Read the model definition and answer for the solid it produces. Units are mm, in the model's axes. A direction names the side the tool comes from. Give positions to 0.01 mm unless a question says otherwise; leave off trailing zeros. Order: outer loops, then holes, each group sorted by start corner. A loop starts at its lowest first (then second) coordinate and runs counter-clockwise, first axis right, second up.
Item 1: A cutting plane is placed at A-A (x = 0). Write down the section's boundary in (y, z), plus the area to 4 significant figures.
Item 2: A cutting plane is placed at B-B (y = -63). Write down the section's boundary in (x, z), plus the area to 3 significant figures.
Item 3: Which of the six approach directions +Z, -Z, +X, -X, +Y, -Y give full straight-line access (tool end or side, diameter ignored) to faces 4 (the face through (0, -37, 23.65)), 5 (the face through (0, -75, 26)), 6 (the face through (-15.81, 1.77, -14.75))?
Item 4: The mould has two halves that part along X. Classify faces 1 (the face through (-0.54, 2.46, 2.44)), 2 (the face through (27.5, -14, 25)), 3 (the face through (0, -34, 28.65)): +X half, -X half, draft (parallel to the pull), parting line (faces both ways), or undercut.
Item 5: A cutting plane is placed at D-D (y = -47.5). Write down the section's boundary in (x, z).
Item 6: Find the intervals of material crossed by line 1 along X through (y, z) = (1, -16); line 2 along Y through (x, z) = (15.5, 24.95); line 3 along Z through (x, y) = (15.5, 1), in increasing order.
Item 7: Given pin 1 Ø16.5 at (x, y) = (6, -36) entering from -Z; pin 2 Ø15.5 at (x, z) = (-7, -3.5) entering from -Y; pin 3 Ø4.5 at (x, y) = (0, -47.5) entering from -Z, each flat-ended and moving along its own axis, determine where each tip first touches the part or whether it passes through.
Item 8: A cutting plane is placed at C-C (z = 0). Write down the section's boundary in (x, y).
from build123d import *

# Parameters (mm, degrees)
SKETCH1_W                                         = 55
SKETCH1_H                                         = 57.3
SKETCH1_R                                         = 2.5
BOSS_EXTRUDE1_DEPTH                               = 5
SKETCH2_W                                         = 55
SKETCH2_H                                         = 5
BOSS_EXTRUDE2_DEPTH                               = 75
CUT_EXTRUDE1_REACH                                = 59.3
CUT_EXTRUDE2_REACH                                = 7
CUT_EXTRUDE3_REACH                                = 59.3
SKETCH5_R                                         = 2.5
CUT_EXTRUDE4_REACH                                = 59.3
SKETCH6_R                                         = 2.5
CUT_EXTRUDE5_REACH                                = 7
CSK_FOR_M2_5_FLAT_HEAD_MACHINE_SCREW1_D           = 2.9
CSK_FOR_M2_5_FLAT_HEAD_MACHINE_SCREW1_DEPTH       = 5
CSK_FOR_M2_5_FLAT_HEAD_MACHINE_SCREW1_CSINK_D     = 5.5
CSK_FOR_M2_5_FLAT_HEAD_MACHINE_SCREW1_CSINK_ANGLE = 90
F_6_40_TAPPED_HOLE1_D                             = 2.8702
F_6_40_TAPPED_HOLE1_DEPTH                         = 3.5
F_6_40_TAPPED_HOLE1_TIP                           = 0.862295074


with BuildPart() as part:
    # Sketch1 → Boss-Extrude1 (new body)
    with BuildSketch(Plane(origin=(0, 0, 0), x_dir=(1, 0, 0), z_dir=(0, 1, 0))):
        Rectangle(SKETCH1_W, SKETCH1_H)
        Circle(SKETCH1_R, mode=Mode.SUBTRACT)
    extrude(amount=BOSS_EXTRUDE1_DEPTH)

    # Sketch2 → Boss-Extrude2 (add)
    with BuildSketch(Plane.XZ):
        with Locations((0, 26.15)):
            Rectangle(SKETCH2_W, SKETCH2_H)
        with Locations((0, -26.15)):
            Rectangle(SKETCH2_W, SKETCH2_H)
    extrude(amount=BOSS_EXTRUDE2_DEPTH)

    # Sketch3 → Cut-Extrude1 (cut, up to next)
    with BuildSketch(Plane.XY.offset(28.65), mode=Mode.PRIVATE) as cut_extrude1_sk1:
        Polygon((-27.5, -75), (-17.5, -75), (-27.5, -65), align=None)
    cut_extrude1_tool1 = extrude(cut_extrude1_sk1.sketch, amount=-CUT_EXTRUDE1_REACH, mode=Mode.PRIVATE) & part.part
    add(cut_extrude1_tool1.solids().sort_by_distance((-24.166667, -71.666667, 28.65))[0], mode=Mode.SUBTRACT)
    # Sketch3 → Cut-Extrude1 (cut, up to next)
    with BuildSketch(Plane.XY.offset(28.65), mode=Mode.PRIVATE) as cut_extrude1_sk2:
        Polygon((27.5, -75), (27.5, -65), (17.5, -75), align=None)
    cut_extrude1_tool2 = extrude(cut_extrude1_sk2.sketch, amount=-CUT_EXTRUDE1_REACH, mode=Mode.PRIVATE) & part.part
    add(cut_extrude1_tool2.solids().sort_by_distance((24.166667, -71.666667, 28.65))[0], mode=Mode.SUBTRACT)

    # Sketch4 → Cut-Extrude2 (cut, up to next)
    with BuildSketch(Plane.XY.offset(-23.65), mode=Mode.PRIVATE) as cut_extrude2_sk1:
        Polygon((-27.5, -65), (-27.5, -75), (-17.5, -75), align=None)
    cut_extrude2_tool1 = extrude(cut_extrude2_sk1.sketch, amount=-CUT_EXTRUDE2_REACH, mode=Mode.PRIVATE) & part.part
    add(cut_extrude2_tool1.solids().sort_by_distance((-24.166667, -71.666667, -23.65))[0], mode=Mode.SUBTRACT)
    # Sketch4 → Cut-Extrude2 (cut, up to next)
    with BuildSketch(Plane.XY.offset(-23.65), mode=Mode.PRIVATE) as cut_extrude2_sk2:
        Polygon((27.5, -65), (17.5, -75), (27.5, -75), align=None)
    cut_extrude2_tool2 = extrude(cut_extrude2_sk2.sketch, amount=-CUT_EXTRUDE2_REACH, mode=Mode.PRIVATE) & part.part
    add(cut_extrude2_tool2.solids().sort_by_distance((24.166667, -71.666667, -23.65))[0], mode=Mode.SUBTRACT)

    # Sketch5 → Cut-Extrude3 (cut, up to next)
    with BuildSketch(Plane.XY.offset(28.65), mode=Mode.PRIVATE) as cut_extrude3_sk1:
        with Locations((0, -47.5)):
            Circle(SKETCH5_R)
    cut_extrude3_tool1 = extrude(cut_extrude3_sk1.sketch, amount=-CUT_EXTRUDE3_REACH, mode=Mode.PRIVATE) & part.part
    add(cut_extrude3_tool1.solids().sort_by_distance((0, -47.5, 28.65))[0], mode=Mode.SUBTRACT)

    # Sketch6 → Cut-Extrude4 (cut, up to next)
    with BuildSketch(Plane(origin=(0, 0, -28.65), x_dir=(-1, 0, 0), z_dir=(0, 0, -1)), mode=Mode.PRIVATE) as cut_extrude4_sk1:
        with Locations((0, -47.5)):
            Circle(SKETCH6_R)
    cut_extrude4_tool1 = extrude(cut_extrude4_sk1.sketch, amount=-CUT_EXTRUDE4_REACH, mode=Mode.PRIVATE) & part.part
    add(cut_extrude4_tool1.solids().sort_by_distance((0, -47.5, -28.65))[0], mode=Mode.SUBTRACT)

    # Sketch7 → Cut-Extrude5 (cut, up to next)
    with BuildSketch(Plane.XY.offset(-23.65), mode=Mode.PRIVATE) as cut_extrude5_sk1:
        Polygon((-27.5, 0), (27.5, 0), (27.5, -65), (17.5, -75), (-17.5, -75), (-27.5, -65), align=None)
    cut_extrude5_tool1 = extrude(cut_extrude5_sk1.sketch, amount=-CUT_EXTRUDE5_REACH, mode=Mode.PRIVATE) & part.part
    add(cut_extrude5_tool1.solids().sort_by_distance((0, -36.651139, -23.65))[0], mode=Mode.SUBTRACT)

    # CSK for M2.5 Flat Head Machine Screw1
    with Locations(Plane.XY.offset(28.65)):
        with Locations((-15.5, -32), (15.5, -32), (-15.5, -63), (15.5, -63)):
            CounterSinkHole(CSK_FOR_M2_5_FLAT_HEAD_MACHINE_SCREW1_D / 2, CSK_FOR_M2_5_FLAT_HEAD_MACHINE_SCREW1_CSINK_D / 2, depth=CSK_FOR_M2_5_FLAT_HEAD_MACHINE_SCREW1_DEPTH, counter_sink_angle=CSK_FOR_M2_5_FLAT_HEAD_MACHINE_SCREW1_CSINK_ANGLE)

    # #6-40 Tapped Hole1
    with Locations(Plane(origin=(0, 0, 0), x_dir=(-1, 0, 0), z_dir=(0, -1, 0))):
        with Locations((-15.5, 16.15), (15.5, 16.15)):
            Hole(F_6_40_TAPPED_HOLE1_D / 2, depth=F_6_40_TAPPED_HOLE1_DEPTH)
            with Locations((0, 0, -(F_6_40_TAPPED_HOLE1_DEPTH + F_6_40_TAPPED_HOLE1_TIP / 2))):  # 118° drill point
                Cone(0, F_6_40_TAPPED_HOLE1_D / 2, F_6_40_TAPPED_HOLE1_TIP, mode=Mode.SUBTRACT)


solid = part.part
Response values:
1. outline: (-75, 23.65) - (-50, 23.65) - (-50, 28.65) - (-75, 28.65) - close; (-45, 23.65) - (0, 23.65) - (0, 2.5) - (5, 2.5) - (5, 28.65) - (-45, 28.65) - close; (0, -28.65) - (5, -28.65) - (5, -2.5) - (0, -2.5) - close
1. area: 611.5 mm2
2. outline: (-27.5, 23.65) - (-16.95, 23.65) - (-16.95, 27.35) - (-18.25, 28.65) - (-27.5, 28.65) - close; (-14.05, 23.65) - (14.05, 23.65) - (14.05, 27.35) - (12.75, 28.65) - (-12.75, 28.65) - (-14.05, 27.35) - close; (16.95, 23.65) - (27.5, 23.65) - (27.5, 28.65) - (18.25, 28.65) - (16.95, 27.35) - close
2. area: 243 mm2
3. face 4: -Z, +X, -X, -Y
3. face 5: +Z, -Z, +X, -X, -Y
3. face 6: -Y
4. face 1: undercut
4. face 2: +X half
4. face 3: draft
5. outline: (-27.5, 23.65) - (-2.5, 23.65) - (-2.5, 28.65) - (-27.5, 28.65) - close; (2.5, 23.65) - (27.5, 23.65) - (27.5, 28.65) - (2.5, 28.65) - close
6. line 1: x = -27.5 to -16.93, -14.07 to 14.07, 16.93 to 27.5
6. line 2: y = -75 to -64.45, -61.55 to -33.45, -30.55 to 5
6. line 3: z = -28.65 to -17.59, -14.71 to 28.65
7. pin 1: stops at z = 23.65
7. pin 2: stops at y = 0
7. pin 3: passes through
8. outline: (-27.5, 0) - (-2.5, 0) - (-2.5, 5) - (-27.5, 5) - close; (2.5, 0) - (27.5, 0) - (27.5, 5) - (2.5, 5) - close
